```python
from build123d import *

# Parameters (mm, degrees)
SKETCH1_W           = 4
SKETCH1_H           = 10
SKETCH1_W_2         = 200
SKETCH1_H_2         = 85
SKETCH1_R           = 3
SKETCH1_R_2         = 7.5
SKETCH1_R_3         = 6
BOSS_EXTRUDE4_DEPTH = 4


with BuildPart() as part:
    # Sketch1 → Boss-Extrude4 (new body)
    # profile 1 of 9: a face of its own
    with BuildSketch(Plane(origin=(0, 0, 0), x_dir=(1, 0, 0), z_dir=(0, 1, 0))):
        with Locations((-2, 80)):
            Rectangle(SKETCH1_W, SKETCH1_H)
    # profile 2 of 9: a face of its own
    with BuildSketch(Plane(origin=(0, 0, 0), x_dir=(1, 0, 0), z_dir=(0, 1, 0))):
        with Locations((-2, 55)):
            Rectangle(SKETCH1_W, SKETCH1_H)
    # profile 3 of 9: a face of its own
    with BuildSketch(Plane(origin=(0, 0, 0), x_dir=(1, 0, 0), z_dir=(0, 1, 0))):
        with Locations((-2, 30)):
            Rectangle(SKETCH1_W, SKETCH1_H)
    # profile 4 of 9: a face of its own
    with BuildSketch(Plane(origin=(0, 0, 0), x_dir=(1, 0, 0), z_dir=(0, 1, 0))):
        with Locations((-2, 5)):
            Rectangle(SKETCH1_W, SKETCH1_H)
    # profile 5 of 9: a face of its own
    with BuildSketch(Plane(origin=(0, 0, 0), x_dir=(1, 0, 0), z_dir=(0, 1, 0))):
        with Locations((202, 5)):
            Rectangle(SKETCH1_W, SKETCH1_H)
    # profile 6 of 9: a face of its own
    with BuildSketch(Plane(origin=(0, 0, 0), x_dir=(1, 0, 0), z_dir=(0, 1, 0))):
        with Locations((202, 30)):
            Rectangle(SKETCH1_W, SKETCH1_H)
    # profile 7 of 9: a face of its own
    with BuildSketch(Plane(origin=(0, 0, 0), x_dir=(1, 0, 0), z_dir=(0, 1, 0))):
        with Locations((202, 55)):
            Rectangle(SKETCH1_W, SKETCH1_H)
    # profile 8 of 9: a face of its own
    with BuildSketch(Plane(origin=(0, 0, 0), x_dir=(1, 0, 0), z_dir=(0, 1, 0))):
        with Locations((202, 80)):
            Rectangle(SKETCH1_W, SKETCH1_H)
    # profile 9 of 9: a face of its own
    with BuildSketch(Plane(origin=(0, 0, 0), x_dir=(1, 0, 0), z_dir=(0, 1, 0))):
        with Locations((100, 42.5)):
            Rectangle(SKETCH1_W_2, SKETCH1_H_2)
        with Locations(Location((60, 60, 0), (0, 0, 270))):
            Circle(SKETCH1_R, mode=Mode.SUBTRACT)
        with Locations(Location((60, 45, 0), (0, 0, 270))):
            Circle(SKETCH1_R_2, mode=Mode.SUBTRACT)
        with Locations(Location((30, 45, 0), (0, 0, 270))):
            Circle(SKETCH1_R_3, mode=Mode.SUBTRACT)
    extrude(amount=BOSS_EXTRUDE4_DEPTH)


solid = part.part
```
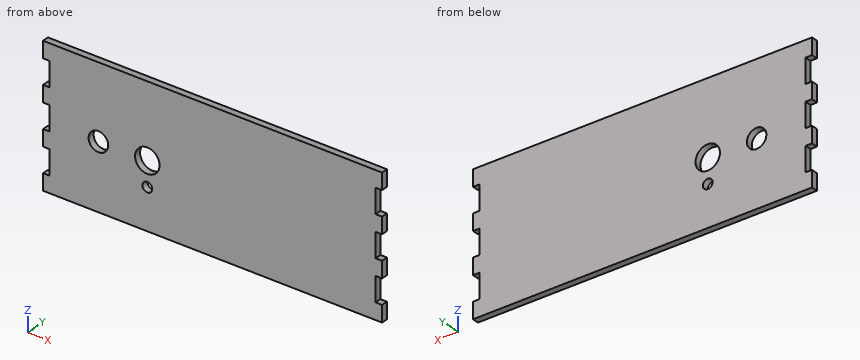
The model under review builds one solid part; all positions refer to its coordinate system, in mm. Give positions to 0.01 mm unless a question says otherwise; leave off trailing zeros. Order: outer loops, then holes, each group sorted by start corner. A loop starts at its lowest first (then second) coordinate and runs counter-clockwise, first axis right, second up. Notation, with made-up numbers: (9, 28.25) - (53, 28.25) arc R24 ccw to (53, 58.25) - close; hole circle Ø9 at (-9.5, 56.25). An arc over 180 degrees is marked (long way). Use CSV: the item, a comma, the result in double quotes. Start each with the question number.
Q1. To check wall thickness, follow line 1 along X through (y, z) = (2.05, -45); line 2 along X through (y, z) = (3.15, -48); line 3 along X through (y, z) = (1, -61). State the ranges of each line that lie inside material, in increasing order. Write a range as [from, to].
Q2. We need section A-A, the plane z = -45. Write out the cut boundary in (x, y), and give its area (3 significant figures).
Q3. Clearance check with flat-ended pins moving along their axes: pin 1 Ø2 at (y, z) = (2.5, -46) entering from +X; pin 2 Ø2 at (y, z) = (2.5, -71) entering from -X. State where each tip first meets the part, or that it passes through.
Q4. We need section B-B, the plane x = 30. Write out the cut boundary in (y, z), and give its area (3 significant figures).
Q5. We need section C-C, the plane y = 1.8. State how many separate pieces and enclosed holes the cut face has, and give its area (3 significant figures).
Q6. We need section D-D, the plane x = 60. Write out the cut boundary in (y, z), and give its area (3 significant figures).
Outcome:
1,line 1,"x = [0, 24], [36, 52.5], [67.5, 200]"
1,line 2,"x = [0, 24.8], [35.2, 53.13], [66.87, 200]"
1,line 3,"x = [0, 57.17], [62.83, 200]"
2,outline,"(0, 0) - (24, 0) - (24, 4) - (0, 4) - close; (36, 0) - (52.5, 0) - (52.5, 4) - (36, 4) - close; (67.5, 0) - (200, 0) - (200, 4) - (67.5, 4) - close"
2,area,"692 mm^2"
3,pin 1,"stops at x = 200"
3,pin 2,"stops at x = 0"
4,outline,"(0, -85) - (4, -85) - (4, -51) - (0, -51) - close; (0, -39) - (4, -39) - (4, 0) - (0, 0) - close"
4,area,"292 mm^2"
5,separate pieces,"1"
5,enclosed holes,"3"
5,area,"17,000 mm^2"
6,outline,"(0, -85) - (4, -85) - (4, -63) - (0, -63) - close; (0, -57) - (4, -57) - (4, -52.5) - (0, -52.5) - close; (0, -37.5) - (4, -37.5) - (4, 0) - (0, 0) - close"
6,area,"256 mm^2"
